Part model, mm, in its own coordinate system. Face numbers are marked on the shaded views. A direction names the side the tool comes from. Round coordinates to 2 decimals unless told otherwise and drop trailing zeros. Loops run counter-clockwise (first coordinate to the right, second up) from the corner with the lowest first, then second, coordinate; pieces in that order, holes last. Notation, with made-up numbers: (86, 61) -> (132, 61) arc R17 cw to (132, 86) -> close; hole circle Ø7 at (48, 64.5). An arc over 180 degrees is marked (long way). Answer as CSV lines item,"result".
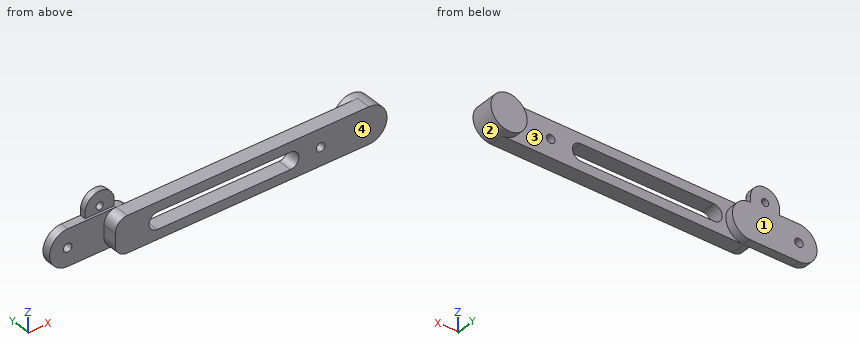
Autodesk Inventor part; units mm, degrees
ref_plane "YZ Plane" through (0, 0, 0) normal (1, 0, 0) x (0, 1, 0)
ref_plane "XZ Plane" through (0, 0, 0) normal (0, 1, 0) x (-1, 0, 0)
ref_plane "XY Plane" through (0, 0, 0) normal (0, 0, 1) x (1, 0, 0)
sketch "Boceto1" plane through (0, 0, 0) normal (0, 1, 0) x (-1, 0, 0)
  arc A0 (0, 7.5) -> (0, -7.5) centre (0, 0) ccw
  circle A1 centre (20, 0) radius 1.75
  arc A2 (32.5, 3.5) -> (32.5, -3.5) centre (32.5, 0) ccw
  arc A3 (87.5, -3.5) -> (87.5, 3.5) centre (87.5, 0) ccw
  line L0 (100, 7.5) -> (0, 7.5)
  line L1 (100, -7.5) -> (0, -7.5)
  arc A4 (105, 2.5) -> (100, 7.5) centre (100, 2.5) ccw
  arc A5 (100, -7.5) -> (105, -2.5) centre (100, -2.5) ccw
  circle A6 centre (120, 0) radius 1.75
  arc A7 (120, -7.5) -> (120, 7.5) centre (120, 0) ccw
  line L2 (120, 7.5) -> (100, 7.5)
  line L3 (120, -7.5) -> (100, -7.5)
  line L4 (105, -2.5) -> (105, 2.5)
  line L5 (100, -7.5) -> (100, -10.5)
  circle A8 centre (103, -10.5) radius 1.5
  arc A9 (100, -10.5) -> (106, -10.5) centre (103, -10.5) ccw
  line L6 (106, -10.5) -> (106, -7.5)
  circle A10 centre (0, 0) radius 7.5
  line L7 (87.5, 3.5) -> (32.5, 3.5)
  line L8 (87.5, -3.5) -> (32.5, -3.5)
  point P0 (0, -7.5)
  point P1 (0, 7.5)
  point P2 (0, 7.5)
  point P3 (0, -7.5)
  dimension "d0" = 15
  dimension "d2" = 3.5
  dimension "d6" = 7
  dimension "d7" = 7
  dimension "d16" = 3.5
  dimension "d18" = 3
  dimension "d20" = 3
  dimension "d22" = 3
  dimension "d23" = 15
  dimension "d24" = 55
  dimension "d25" = 55
extrude "Extrusión1" add sketch "Boceto1" along normal blind 9.5 contours A10 A0
extrude "Extrusión2" add sketch "Boceto1" along normal blind 6 contours L0 A4 L4 A5 L1 A10
sketch "Boceto2" plane through (0, 6, 0) normal (0, 1, 0) x (1, 0, 0)
  line L0 (-100, -7.5) -> (0, -7.5)
  arc A0 (0, 7.5) -> (0, -7.5) centre (0, 0) ccw
  line L1 (0, 7.5) -> (-100, 7.5)
  arc A1 (-100, 7.5) -> (-105, 2.5) centre (-100, 2.5) ccw
  line L2 (-105, 2.5) -> (-105, -2.5)
  arc A2 (-105, -2.5) -> (-100, -7.5) centre (-100, -2.5) ccw
  circle A3 centre (-20, 0) radius 1.75
  line L3 (-87.5, 3.5) -> (-32.5, 3.5)
  arc A4 (-32.5, -3.5) -> (-32.5, 3.5) centre (-32.5, 0) ccw
  line L4 (-32.5, -3.5) -> (-87.5, -3.5)
  arc A5 (-87.5, 3.5) -> (-87.5, -3.5) centre (-87.5, 0) ccw
  arc A6 (-120, 7.5) -> (-120, -7.5) centre (-120, 0) ccw
  line L5 (-120, -7.5) -> (-100, -7.5)
  line L6 (-120, 7.5) -> (-100, 7.5)
  arc A7 (-100, -7.5) -> (-100, 7.5) centre (-100, 0) ccw
  line L7 (-100, -7.5) -> (0, -7.5)
  line L8 (-100, -7.5) -> (-100, -10.5)
  circle A8 centre (-103, -10.5) radius 1.5
  arc A9 (-106, -10.5) -> (-100, -10.5) centre (-103, -10.5) ccw
  line L9 (-106, -10.5) -> (-106, -7.5)
  circle A10 centre (-120, 0) radius 1.75
  dimension "d31" = 15
  dimension "d32" = 20
  dimension "d33" = 20
  dimension "d35" = 3
  dimension "d39" = 3
  dimension "d40" = 3.5
extrude "Extrusión3" add sketch "Boceto2" along normal blind 3.5 contours L5 A6 L6 A1 L2 A2 | A2 L2 A1 A7
sketch "Boceto3" plane through (0, 9.5, 0) normal (0, 1, 0) x (1, 0, 0)
  line L0 (-105, 2.5) -> (-105, -2.5)
  line L1 (-120, -7.5) -> (-100, -7.5)
  arc A0 (-100, -7.5) -> (-100, 7.5) centre (-100, 0) ccw
  line L2 (-100, 7.5) -> (-120, 7.5)
  arc A1 (-120, 7.5) -> (-120, -7.5) centre (-120, 0) ccw
  circle A2 centre (-120, 0) radius 1.75
  arc A3 (-100, -7.5) -> (-100, 7.5) centre (-100, 0) ccw
  line L3 (-100, -7.5) -> (0, -7.5)
  arc A4 (0, 7.5) -> (0, -7.5) centre (0, 0) ccw
  line L4 (0, 7.5) -> (-100, 7.5)
  circle A5 centre (-20, 0) radius 1.75
  line L5 (-87.5, 3.5) -> (-32.5, 3.5)
  arc A6 (-32.5, -3.5) -> (-32.5, 3.5) centre (-32.5, 0) ccw
  line L6 (-32.5, -3.5) -> (-87.5, -3.5)
  arc A7 (-87.5, 3.5) -> (-87.5, -3.5) centre (-87.5, 0) ccw
  line L7 (-100, -7.5) -> (-100, -10.4769)
  line L8 (-120, -7.5) -> (-100, -7.5)
  line L9 (-106, -7.5) -> (-100, -7.5)
  line L10 (-111.9608, -7.5) -> (-111.9608, -10.5)
  arc A8 (-111.9608, -10.5) -> (-100, -10.4769) centre (-105.9813, -10.0037) ccw
  circle A9 centre (-105.9813, -10.0037) radius 1.5
  dimension "d52" = 3
  dimension "d53" = 6
  dimension "d54" = 3
extrude "Extrusión4" add sketch "Boceto3" against normal blind 2.5 contours L1 L7 A8 L10
properties part number "pieza4parte3"
Q1. Saw through at D-D, the plane z = 6. Write the cut outline in (x, y).
Geometry results:
outline,"(-124.5, 6) -> (-103.57, 6) -> (-103.57, 0) -> (4.5, 0) -> (4.5, 9.5) -> (-4.5, 9.5) -> (-4.5, 6) -> (-95.5, 6) -> (-95.5, 9.5) -> (-124.5, 9.5) -> close"
Q2. Saw through at C-C, the plane x = -20. Write the cut outline in (y, z), then the cut area to 3 significant figures.
Geometry results:
outline,"(0, -7.5) -> (6, -7.5) -> (6, -1.75) -> (0, -1.75) -> close; (0, 1.75) -> (6, 1.75) -> (6, 7.5) -> (0, 7.5) -> close"
area,"69.0 mm2"
Q3. Saw through at A-A, the plane x = -37. Write the cut outline in (y, z).
Geometry results:
outline,"(0, -7.5) -> (6, -7.5) -> (6, -3.5) -> (0, -3.5) -> close; (0, 3.5) -> (6, 3.5) -> (6, 7.5) -> (0, 7.5) -> close"
Q4. Which spindle directions (+Z, -Z, +X, -X, +Y, -Y) get a long thin tool onto all of the face, cutting with end or side? Do the marked faces 1 and 2. Say none if no direction does.
Geometry results:
face 1,"+Z, -Z, +X, -X, +Y"
face 2,"+Y"
Q5. Drill centre lines: line 1 along X through (y, z) = (9, 0.25); line 2 along Z through (x, y) = (-60, 2.25); line 3 along X through (y, z) = (3.5, -1.5). Where is each one in solid material? Low to high.
Geometry results:
line 1,"-127.5 to -121.73, -118.27 to -92.5, -7.5 to 7.5"
line 2,"-7.5 to -3.5, 3.5 to 7.5"
line 3,"-105 to -90.66, -29.34 to -20.9, -19.1 to 7.35"
Q6. Saw through at B-B, the plane y = 4.5. Write the cut outline in (x, z), then the cut area to 3 significant figures.
Geometry results:
outline,"(-105, -2.5) arc R5 ccw to (-100, -7.5) -> (0, -7.5) arc R7.5 ccw to (0, 7.5) -> (-100, 7.5) arc R5 ccw to (-105, 2.5) -> close; hole (-87.5, -3.5) -> (-32.5, -3.5) arc R3.5 ccw to (-32.5, 3.5) -> (-87.5, 3.5) arc R3.5 ccw to start; hole circle Ø3.5 at (-20, 0)"
area,"1,220 mm2"
Q7. Drop flat-ended pins along their axis: P1, Ø2.5, axis at x = -108, z = 13.5, coming from the -Y side; P2, Ø3, axis at x = -108.5, y = 8, coming from the +Z side; P3, Ø3, axis at y = 6, z = 6.5, coming from the -X side. Give the stop position or say it passes through.
Geometry results:
P1,"y = 7"
P2,"z = 15.92"
P3,"x = -125.59"
Q8. Two-plate mould, pull along X, no slides. Class the marked faces 3 and 4: pulls with the +X half, pulls with the -X half, needs draft (parallel to the pull), parting line crosses it, or undercut.
Geometry results:
face 3,"undercut"
face 4,"needs draft"
